Job drawing, mm, ordinate dimensions from the low corner. One solid piece. A direction names the side the tool comes from. Give positions to 0.01 mm unless a question says otherwise; leave off trailing zeros. Write each loop counter-clockwise with the first axis right and the second up, starting at its lowest first coordinate (ties: lowest second). Pieces come first, ordered by that corner, then holes. Notation, with made-up numbers: (-30.5, 22.25) -> (-11.5, 22.25) arc R10 ccw to (-11.5, 31.25) -> close; hole circle Ø3 at (-27.5, 50). An arc over 180 degrees is marked (long way). One line per question, with ' | ' between items. Start each with the question number.
(1) Pin check, flat tips, straight feed: P1, Ø1.5, axis at x = 13.5, y = 4.5, coming from the -Z side; P2, Ø1.5, axis at x = 11, y = 4, coming from the -Z side; P3, Ø2.5, axis at y = 2, z = 19, coming from the +X side. Stop position of each tip, or through.
(2) Band-saw the part on A-A, the plane x = 17. Give the cut face in (y, z), and give its area (3 significant figures).
(3) Tool access for the marked faces 1, 2 and 3: list every direction of +Z, -Z, +X, -X, +Y, -Y with a clear straight run to the whole face (end or side of a thin tool).
(4) Band-saw the part on B-B, the plane z = 9.5. Give the cut face in (x, y).
(5) Drill centre lines: probe 1 along X at (y, z) = (2.4, 10); probe 2 along X at (y, z) = (3.55, 13.5) (1 decimal); probe 3 along X at (y, z) = (3.45, 24). Where is each one in solid material? Low to high. Write a range as from..to.
(6) Pull direction Z, two halves, no side cores. Call the marked faces 4, 5, 6 and 7: released by +Z, released by -Z, zero draft, split by the parting line, or undercut.
(7) Band-saw the part on D-D, the plane x = 4.25. Give the cut face in (y, z).
(8) Band-saw the part on C-C, the plane y = 2.9. Give the cut face in (x, z).
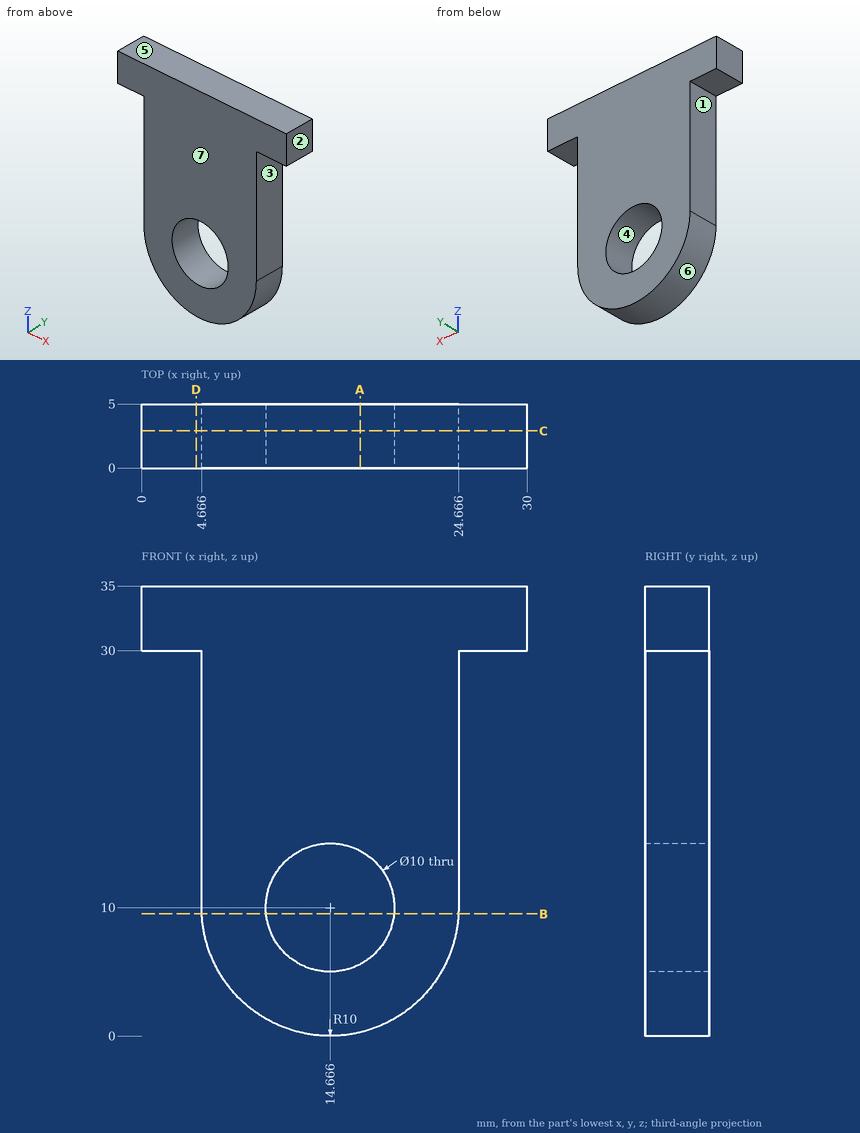
Results:
1) P1: stops at z = 0.01 | P2: stops at z = 0.43 | P3: stops at x = 24.67
2) outline: (0, 0.28) -> (5, 0.28) -> (5, 5.58) -> (0, 5.58) -> close; (0, 14.42) -> (5, 14.42) -> (5, 35) -> (0, 35) -> close | area: 129 mm²
3) face 1: -Z, -X, +Y, -Y | face 2: +Z, -Z, +X, +Y, -Y | face 3: -Z, +X, +Y, -Y
4) outline: (4.68, 0) -> (9.69, 0) -> (9.69, 5) -> (4.68, 5) -> close; (19.64, 0) -> (24.65, 0) -> (24.65, 5) -> (19.64, 5) -> close
5) probe 1: x = 4.67..9.67, 19.67..24.67 | probe 2: x = 4.7..11.1, 18.2..24.7 | probe 3: x = 4.67..24.67
6) face 4: undercut | face 5: released by +Z | face 6: released by -Z | face 7: zero draft
7) outline: (0, 30) -> (5, 30) -> (5, 35) -> (0, 35) -> close
8) outline: (0, 30) -> (4.67, 30) -> (4.67, 10) arc R10 ccw to (24.67, 10) -> (24.67, 30) -> (30, 30) -> (30, 35) -> (0, 35) -> close; hole circle Ø10 at (14.67, 10)
